CAD build for the part. Positions are in the model's coordinates, mm. A direction names the side the tool comes from. Round coordinates to 2 decimals unless told otherwise and drop trailing zeros. Loops run counter-clockwise (first coordinate to the right, second up) from the corner with the lowest first, then second, coordinate; pieces in that order, holes last. Notation, with made-up numbers: (67.5, 20) - (109.5, 20) arc R10 ccw to (109.5, 29) - close; hole circle Ø5 at (64, 12). An arc over 180 degrees is marked (long way). Use one line per item in the form item = value.
from build123d import *

# Parameters (mm, degrees)
F1_DEPTH = 150
F2_T     = -12


# Not quite as in the source:
# - a shell that OpenCascade refuses in one call is made with other operations: the cavity is built on its own and cut out


with BuildPart() as f1:
    # F0 (on Top) → F1 (new body)
    with BuildSketch(Plane.XY):
        Polygon((150, 150), (-150, 150), (-150, -150), (0, -150), (0, 0), (150, 0), align=None)
    extrude(amount=-F1_DEPTH)

    # F2: a shell. OpenCascade refuses it in one call, so the cavity is built on its own and cut out:
    # the body offset inwards by the wall thickness, plus a prism from it out through each open face.
    f2_core = offset(f1.part, amount=F2_T, kind=Kind.INTERSECTION, mode=Mode.PRIVATE)
    f2_exits = [f2_core.faces().sort_by_distance(p)[0] for p in [
        (-12, -63, -75),
    ]]
    add(f2_core, mode=Mode.SUBTRACT)
    extrude(f2_exits, amount=-F2_T, mode=Mode.SUBTRACT)


solid = f1.part
1) Flat gauge pins, fed straight in: pin 1 (1 mm diameter, centred on x = -35, y = -53, fed in from +Z); pin 2 (5 mm diameter, centred on y = -74, z = -134.5, fed in from +X); pin 3 (2 mm diameter, centred on x = 89, z = -108.5, fed in from -Y). Where does each tip first touch, or does it go through?
Report:
pin_1 = 0
pin_2 = -138
pin_3 = 0
2) Two-plate mould, pull along Z, no slides. Class faces 6 (the flat face through (0, 6, -74)), 7 (the flat face through (-35, 35, 0)), 8 (the flat face through (-150, 2, -74)), 9 (the flat face through (2, 138, -74)): +Z half, -Z half, draft (parallel to the pull), parting line (faces both ways), or undercut.
Report:
face_6 = undercut
face_7 = +Z half
face_8 = draft
face_9 = undercut
3) Drill centre lines: probe 1 along Z at (x, y) = (-65, 57.5); probe 2 along X at (y, z) = (123, -106.5); probe 3 along Y at (x, z) = (102, -90.5). Where is each one in solid material? Low to high.
Report:
probe_1 = -150 to -138, -12 to 0
probe_2 = -150 to -138, 138 to 150
probe_3 = 0 to 12, 138 to 150
4) Slice it at D-D (z = -28.5). Write the cut outline in (x, y).
Report:
outline = (-150, -150) - (0, -150) - (0, -138) - (-138, -138) - (-138, 138) - (138, 138) - (138, 12) - (0, 12) - (0, 0) - (150, 0) - (150, 150) - (-150, 150) - close
5) Slice it at A-A (x = 91). Write the cut outline in (y, z), plus the area to 3 significant figures.
Report:
outline = (0, -150) - (150, -150) - (150, 0) - (0, 0) - close; hole (12, -138) - (138, -138) - (138, -12) - (12, -12) - close
area = 6,620 mm^2
6) Slice it at B-B (y = -45). Write the cut outline in (x, z), plus the area to 3 significant figures.
Report:
outline = (-150, -150) - (0, -150) - (0, -138) - (-138, -138) - (-138, -12) - (0, -12) - (0, 0) - (-150, 0) - close
area = 5,110 mm^2
7) Slice it at C-C (y = 62.5). Write the cut outline in (x, z).
Report:
outline = (-150, -150) - (150, -150) - (150, 0) - (-150, 0) - close; hole (-138, -138) - (138, -138) - (138, -12) - (-138, -12) - close
8) Tool access for faces 1 (the flat face through (-35, 35, -150)), 2 (the flat face through (-33, 33, -138)), 3 (the flat face through (2, 150, -74)), 4 (the flat face through (74, 0, -74)), 5 (the flat face through (-70, -138, -76)): list every direction of +Z, -Z, +X, -X, +Y, -Y with a clear straight run to the whole face (end or side of a thin tool).
Report:
face_1 = -Z, +X, -X, +Y, -Y
face_2 = none
face_3 = +Z, -Z, +X, -X, +Y
face_4 = +Z, -Z, +X, -Y
face_5 = +X
